The listing builds one solid part. Answer for the finished solid, in the listing's coordinates (mm). A direction names the side the tool comes from. Coordinates: 2 decimals unless noted, no trailing zeros. Order: outer loops, then holes, each group sorted by start corner. A loop starts at its lowest first (then second) coordinate and runs counter-clockwise, first axis right, second up. Notation, with made-up numbers: (80, -21) -> (84, -21) arc R24 cw to (84, 0) -> close; hole circle Ø4 at (34, -7.75). An arc over 180 degrees is marked (long way). Answer in a Markdown table with one row per item.
```python
from build123d import *

# Parameters (mm, degrees)
BOSS_EXTRUDE1_DEPTH = 30
FILLET1_R           = 2
FILLET2_R           = 10
SKETCH2_R           = 4.5
CUT_EXTRUDE1_DEPTH  = 31


with BuildPart() as part:
    # Sketch1 → Boss-Extrude1 (new body)
    with BuildSketch(Plane.XY):
        Polygon((-56.826553722, 0), (0, 90), (56.826553722, 0), (45, 0), (0, 71.26949876), (-45, 0), align=None)
    extrude(amount=BOSS_EXTRUDE1_DEPTH)

    # Fillet1
    fillet1_edges = [part.edges().sort_by_distance(p)[0] for p in [
        (0, 90, 15),
    ]]
    fillet(fillet1_edges, radius=FILLET1_R)

    # Fillet2
    fillet2_edges = [part.edges().sort_by_distance(p)[0] for p in [
        (0, 71.26949876, 15),
    ]]
    fillet(fillet2_edges, radius=FILLET2_R)

    # Sketch2 → Cut-Extrude1 (cut, through all)
    with BuildSketch(Plane.XY.offset(30)):
        with Locations((0, 72.5)):
            Circle(SKETCH2_R)
    extrude(amount=-CUT_EXTRUDE1_DEPTH, mode=Mode.SUBTRACT)


solid = part.part
```
(1) Which of the six approach directions +Z, -Z, +X, -X, +Y, -Y give full straight-line access (tool end or side, diameter ignored) to faces 1 (the flat face through (13, 51, 0)), 2 (the flat face through (-26.5, 29.3, 14.8))?
Check values:
| item | result |
|---|---|
| face 1 | -Z, +X, -X, +Y, -Y |
| face 2 | +Z, -Z, -Y |
(2) A cutting plane is placed at B-B, the plane z = 5.25. Determine the outline of the cut face in (x, y), then the cut area to 3 significant figures.
Check values:
| item | result |
|---|---|
| outline | (-56.83, 0) -> (-45, 0) -> (-8.46, 57.88) arc R10 cw to (8.46, 57.88) -> (45, 0) -> (56.83, 0) -> (1.69, 87.32) arc R2 ccw to (-1.69, 87.32) -> close; hole circle Ø9 at (0, 72.5) |
| area | 1,900 mm² |
(3) A cutting plane is placed at D-D, the plane x = 25. Determine the outline of the cut face in (y, z).
Check values:
| item | result |
|---|---|
| outline | (31.68, 0) -> (50.41, 0) -> (50.41, 30) -> (31.68, 30) -> close |
(4) A cutting plane is placed at A-A, the plane x = 0. Determine the outline of the cut face in (y, z), then the cut area to 3 significant figures.
Check values:
| item | result |
|---|---|
| outline | (62.54, 0) -> (68, 0) -> (68, 30) -> (62.54, 30) -> close; (77, 0) -> (88.25, 0) -> (88.25, 30) -> (77, 30) -> close |
| area | 501 mm² |
(5) Flat-ended cylindrical pins translate along their axes: pin 1 (12 mm diameter, centred on y = 47, z = 3.5, fed in from +X); pin 2 (6 mm diameter, centred on y = 19.5, z = 17, fed in from +X); pin 3 (11.5 mm diameter, centred on x = 0, y = 72.5, fed in from -Z); pin 4 (12 mm diameter, centred on y = 64, z = 21.5, fed in from +X) (3 decimals). Find the tip coordinate at first contact, or state that the pin passes through.
Check values:
| item | result |
|---|---|
| pin 1 | x = 30.94 |
| pin 2 | x = 46.41 |
| pin 3 | z = 0 |
| pin 4 | x = 20.205 |
(6) Find the intervals of material crossed by line 1 along X through (y, z) = (56.5, 22); line 2 along X through (y, z) = (59, 26.75); line 3 along Y through (x, z) = (-31, 6), in increasing order. Write a range as from..to.
Check values:
| item | result |
|---|---|
| line 1 | -21.15..-9.33, 9.33..21.15 |
| line 2 | -19.57..-7.63, 7.63..19.57 |
| line 3 | 22.17..40.9 |
(7) A cutting plane is placed at C-C, the plane y = 22.5. Determine the outline of the cut face in (x, z), then the cut area to 3 significant figures.
Check values:
| item | result |
|---|---|
| outline | (-42.62, 0) -> (-30.79, 0) -> (-30.79, 30) -> (-42.62, 30) -> close; (30.79, 0) -> (42.62, 0) -> (42.62, 30) -> (30.79, 30) -> close |
| area | 710 mm² |
(8) For a pull along X with two mould halves and no side action, classify faces 3 (the flat face through (51, 0, 15)), 4 (the flat face through (26.984, 28.534, 14.79)), 5 (the cylindrical face through (-0.59, 76.96, 15.21)), 6 (the cylindrical face through (-0.028, 88.254, 15.21)) as released by +X, released by -X, zero draft, split by the parting line, or undercut.
Check values:
| item | result |
|---|---|
| face 3 | zero draft |
| face 4 | undercut |
| face 5 | undercut |
| face 6 | split by the parting line |
